Geometry check sheet. Reference: the model listing, model coordinates, mm. Give positions to 0.01 mm unless a question says otherwise; leave off trailing zeros. Loops run counter-clockwise (first coordinate to the right, second up) from the corner with the lowest first, then second, coordinate; pieces in that order, holes last. Notation, with made-up numbers: (18, 15.25) -> (68, 15.25) arc R27 ccw to (68, 37.25) -> close; hole circle Ø6 at (40, -7.75). An arc over 180 degrees is marked (long way). Answer as a JSON object with one key per item and string values.
from build123d import *

# Parameters (mm, degrees)
SKETCH1_W           = 43.93
SKETCH1_H           = 15
BOSS_EXTRUDE1_DEPTH = 3
CUT_EXTRUDE1_START  = -4
SKETCH2_R           = 3.9
CUT_EXTRUDE1_DEPTH  = 5


with BuildPart() as part:
    # Sketch1 → Boss-Extrude1 (new body)
    with BuildSketch(Plane(origin=(0, 0, 0), x_dir=(1, 0, 0), z_dir=(0, 1, 0))):
        Rectangle(SKETCH1_W, SKETCH1_H)
    extrude(amount=BOSS_EXTRUDE1_DEPTH)

    # Sketch2 → Cut-Extrude1 (cut)
    with BuildSketch(Plane(origin=(0, 3, 0), x_dir=(1, 0, 0), z_dir=(0, 1, 0)).offset(CUT_EXTRUDE1_START)):
        with Locations((-10, 0)):
            Circle(SKETCH2_R)
    cut_extrude1 = extrude(amount=CUT_EXTRUDE1_DEPTH, mode=Mode.SUBTRACT)

    # Mirror1: Cut-Extrude1 across plane
    add(cut_extrude1.mirror(Plane(origin=(0, 0, 0), x_dir=(0, 0, 1), z_dir=(1, 0, 0))), mode=Mode.SUBTRACT)


solid = part.part
1) Section check C-C on y = 0.7. Record the cut outline in (x, z) (3 decimals).
Geometry check:
{"outline": "(-21.965, -7.5) -> (21.965, -7.5) -> (21.965, 7.5) -> (-21.965, 7.5) -> close; hole circle Ø7.8 at (-10, 0); hole circle Ø7.8 at (10, 0)"}
2) Section check A-A on z = 0. Record the cut outline in (x, y) (3 decimals).
Geometry check:
{"outline": "(-21.965, 0) -> (-13.9, 0) -> (-13.9, 3) -> (-21.965, 3) -> close; (-6.1, 0) -> (6.1, 0) -> (6.1, 3) -> (-6.1, 3) -> close; (13.9, 0) -> (21.965, 0) -> (21.965, 3) -> (13.9, 3) -> close"}
3) Section check B-B on x = -10. Record the cut outline in (y, z), plus the area to 3 significant figures.
Geometry check:
{"outline": "(0, -7.5) -> (3, -7.5) -> (3, -3.9) -> (0, -3.9) -> close; (0, 3.9) -> (3, 3.9) -> (3, 7.5) -> (0, 7.5) -> close", "area": "21.6 mm2"}
4) Material ranges on line 1 along X through (y, z) = (0.85, -0.25) (3 decimals); line 2 along X through (y, z) = (2.15, -3.5) (3 decimals); line 3 along Z through (x, y) = (-10, 1.05), recorded low to high. Write a range as from..to.
Geometry check:
{"line 1": "x = -21.965..-13.892, -6.108..6.108, 13.892..21.965", "line 2": "x = -21.965..-11.72, -8.28..8.28, 11.72..21.965", "line 3": "z = -7.5..-3.9, 3.9..7.5"}
5) Section check D-D on x = 11. Record the cut outline in (y, z).
Geometry check:
{"outline": "(0, -7.5) -> (3, -7.5) -> (3, -3.77) -> (0, -3.77) -> close; (0, 3.77) -> (3, 3.77) -> (3, 7.5) -> (0, 7.5) -> close"}
6) Depth check by flat-ended pin: P1, Ø6, axis at x = -10, z = 0, coming from the -Y side. Enter the tip coordinate at first touch or a pass-through.
Geometry check:
{"P1": "passes through"}
